```python
from build123d import *

# Parameters (mm, degrees)
F0_R     = 25
F1_DEPTH = 1000
F2_R     = 20
F3_DEPTH = 1000.001
F4_R     = 10
F5_DEPTH = 25.4


with BuildPart() as f1:
    # F0 (on Front) → F1 (new body)
    with BuildSketch(Plane.XZ):
        Circle(F0_R)
    extrude(amount=-F1_DEPTH)

    # F2 (on Front) → F3 (cut, through all)
    with BuildSketch(Plane.XZ):
        Circle(F2_R)
    extrude(amount=-F3_DEPTH, mode=Mode.SUBTRACT)

    # F4 (on Top) → F5 (cut)
    with BuildSketch(Plane.XY):
        with Locations((0, 100)):
            Circle(F4_R)
    extrude(amount=F5_DEPTH, mode=Mode.SUBTRACT)


solid = f1.part
```
Here's how the part is built. I have some questions about the finished solid (model axes, mm). Coordinates: 2 decimals unless noted, no trailing zeros. Write each loop counter-clockwise with the first axis right and the second up, starting at its lowest first coordinate (ties: lowest second). Pieces come first, ordered by that corner, then holes. Notation, with made-up numbers: (-33, 16.5) -> (23, 16.5) arc R14 cw to (23, 28.5) -> close; hole circle Ø7 at (-9.75, 18.25). An arc over 180 degrees is marked (long way). Use a Markdown table: item, result. Add a question column.
(1) If we section it at A-A, the plane z = 0: Write out the boundary of the cut face in (x, y), and give its area (3 significant figures).
(2) Please list where these lines run through material, in increasing order: line 1 (Z direction, x = 0, y = 505); line 2 (Y direction, x = 0, z = 22); line 3 (X direction, y = 834.5, z = 1.5).
(3) We'd pull the mould along Y, two halves only. Please class faces 1 (the cylindrical face through (23.846, 493, 7.509)), 2 (the flat face through (-11, 1000, 17)), 3 (the cylindrical face through (-10, 100, 21)): +Y half, -Y half, draft (parallel to the pull), parting line (faces both ways), or undercut.
(4) If we section it at B-B, the plane x = 0: Write out the boundary of the cut face in (y, z), and give its area (3 significant figures).
(5) I'm going to push flat-ended pins straight in: P1, Ø10, axis at y = 646, z = -13, coming from the +X side; P2, Ø18, axis at x = 0, y = 100, coming from the +Z side; P3, Ø2, axis at y = 660.5, z = 16, coming from the -X side. Where does each tip first touch, or does it pass through?
(6) If we section it at C-C, the plane y = 119: Write out the boundary of the cut face in (x, z).
Outcome:
| question | item | result |
|---|---|---|
| 1 | outline | (-25, 0) -> (-20, 0) -> (-20, 1000) -> (-25, 1000) -> close; (20, 0) -> (25, 0) -> (25, 1000) -> (20, 1000) -> close |
| 1 | area | 10,000 mm^2 |
| 2 | line 1 | z = -25 to -20, 20 to 25 |
| 2 | line 2 | y = 0 to 90, 110 to 1000 |
| 2 | line 3 | x = -24.95 to -19.94, 19.94 to 24.95 |
| 3 | face 1 | draft |
| 3 | face 2 | +Y half |
| 3 | face 3 | undercut |
| 4 | outline | (0, -25) -> (1000, -25) -> (1000, -20) -> (0, -20) -> close; (0, 20) -> (90, 20) -> (90, 25) -> (0, 25) -> close; (110, 20) -> (1000, 20) -> (1000, 25) -> (110, 25) -> close |
| 4 | area | 9,900 mm^2 |
| 5 | P1 | stops at x = 23.69 |
| 5 | P2 | stops at z = -17.86 |
| 5 | P3 | stops at x = -20 |
| 6 | outline | circle Ø50 at (0, 0); hole circle Ø40 at (0, 0) |
